Could you check a few things on this model? Use its own coordinates, in mm. Face numbers are marked on the shaded views. A direction names the side the tool comes from. Give positions to 0.01 mm unless a question says otherwise; leave off trailing zeros. Write each loop counter-clockwise with the first axis right and the second up, starting at its lowest first coordinate (ties: lowest second). Pieces come first, ordered by that corner, then holes. Notation, with made-up numbers: M 3,-33 L 14,-33 A33 cw 14,4 Z; hole C -19.5,25 d6. An arc over 180 degrees is marked long. One line per item, written item: value.
```python
from build123d import *

# Parameters (mm, degrees)
SKETCH1_W           = 60.96
SKETCH1_H           = 60.96
BOSS_EXTRUDE1_DEPTH = 10
BOSS_EXTRUDE2_DEPTH = 60.96
SKETCH5_W           = 50.8
SKETCH5_H           = 10.16
BOSS_EXTRUDE3_DEPTH = 10.16
SKETCH6_R           = 6.35
CUT_EXTRUDE1_DEPTH  = 8.89


with BuildPart() as part:
    # Sketch1 → Boss-Extrude1 (new body)
    with BuildSketch(Plane(origin=(0, 0, 0), x_dir=(1, 0, 0), z_dir=(0, 1, 0))):
        with Locations((30.48, 30.48)):
            Rectangle(SKETCH1_W, SKETCH1_H)
    extrude(amount=BOSS_EXTRUDE1_DEPTH)

    # Sketch2 → Boss-Extrude2 (add)
    with BuildSketch(Plane(origin=(0, 10, 0), x_dir=(1, 0, 0), z_dir=(0, 1, 0))):
        Polygon((0, 60.96), (10.16, 60.96), (10.16, 10.16), (60.96, 10.16), (60.96, 0), (0, 0), align=None)
    extrude(amount=BOSS_EXTRUDE2_DEPTH)

    # Sketch5 → Boss-Extrude3 (add)
    with BuildSketch(Plane(origin=(10.16, 0, 0), x_dir=(0, 0, -1), z_dir=(1, 0, 0))):
        with Locations((35.56, 65.88)):
            Rectangle(SKETCH5_W, SKETCH5_H)
    extrude(amount=BOSS_EXTRUDE3_DEPTH)

    # Sketch6 → Cut-Extrude1 (cut)
    with BuildSketch(Plane.XZ):
        with Locations((30.48, -30.48)):
            Circle(SKETCH6_R)
    extrude(amount=-CUT_EXTRUDE1_DEPTH, mode=Mode.SUBTRACT)


solid = part.part
```
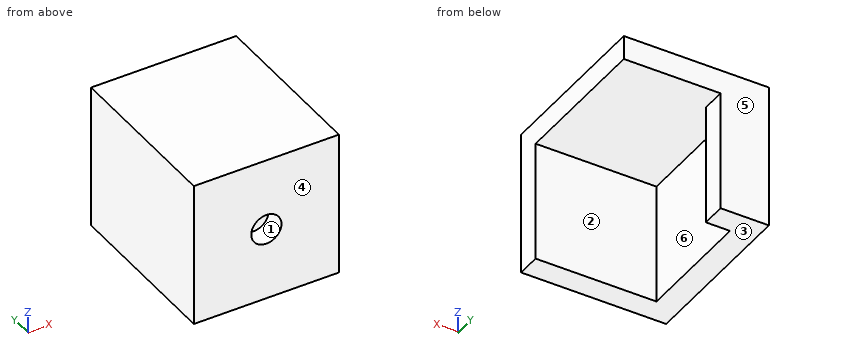
1) If we section it at D-D, the plane x = 12: Write out the boundary of the cut face in (y, z), then the cut area to 3 significant figures.
Outcome:
outline: M 0,-60.96 L 10,-60.96 L 10,-10.16 L 60.8,-10.16 L 60.8,-60.96 L 70.96,-60.96 L 70.96,0 L 0,0 Z
area: 1,750 mm^2
2) We'd pull the mould along Y, two halves only. Please class the marked faces 4, 5 and 6: pulls with the +Y half, pulls with the -Y half, needs draft (parallel to the pull), parting line crosses it, or undercut.
Outcome:
face 4: pulls with the -Y half
face 5: pulls with the +Y half
face 6: undercut
3) If we section it at A-A, the plane x = 30.48: Write out the boundary of the cut face in (y, z), then the cut area to 3 significant figures.
Outcome:
outline: M 0,-60.96 L 10,-60.96 L 10,-10.16 L 70.96,-10.16 L 70.96,0 L 0,0 L 0,-24.13 L 8.89,-24.13 L 8.89,-36.83 L 0,-36.83 Z
area: 1,120 mm^2
4) I'm going to push flat-ended pins straight in: pin 1 (12 mm diameter, centred on x = 28, z = -47, fed in from +Y); pin 2 (3 mm diameter, centred on y = 40, z = -16, fed in from +X); pin 3 (5 mm diameter, centred on y = 62.5, z = -54.5, fed in from +X). Where does each tip first touch, or does it pass through?
Outcome:
pin 1: stops at y = 10
pin 2: stops at x = 10.16
pin 3: stops at x = 20.32
5) If we section it at C-C, the plane z = -48: Write out the boundary of the cut face in (x, y).
Outcome:
outline: M 0,0 L 60.96,0 L 60.96,10 L 10.16,10 L 10.16,60.8 L 20.32,60.8 L 20.32,70.96 L 0,70.96 Z
6) Please list where these lines run through material, in increasing order: L1, parallel to X at y = 6, z = -30; L2, parallel to Z at x = 30, y = 5; L3, parallel to Y at x = 15.5, z = -25. Write a range as from..to.
Outcome:
L1: x = 0..24.15, 36.81..60.96
L2: z = -60.96..-36.81, -24.15..0
L3: y = 0..10, 60.8..70.96
7) If we section it at B-B, the plane y = 26: Write out the boundary of the cut face in (x, z), then the cut area to 3 significant figures.
Outcome:
outline: M 0,-60.96 L 10.16,-60.96 L 10.16,-10.16 L 60.96,-10.16 L 60.96,0 L 0,0 Z
area: 1,140 mm^2
8) On a 3-axis mill with a long thin cutter (end or side, diameter ignored), from which of +Z, -Z, +X, -X, +Y, -Y can I reach the whole of each face in a straight line? I mean the marked faces 1, 2 and 3. Say none if no direction works.
Outcome:
face 1: -Y
face 2: -Z, +X
face 3: -Z, +X, -X, +Y, -Y
